The figure shows three views and two pictorial views of one solid part (mm, origin at its lowest corner). Answer the questions. A direction names the side the tool comes from. Round coordinates to 2 decimals unless told otherwise and drop trailing zeros. Write each loop counter-clockwise with the first axis right and the second up, starting at its lowest first coordinate (ties: lowest second). Pieces come first, ordered by that corner, then holes.
Item 1: A tool of negligible diameter and unlimited length cuts with its end or side. For the marked faces 1 and 2, from which of +Z, -Z, +X, -X, +Y, -Y can it reach the whole face along a straight path? Write none if from no direction.
Item 2: Find section C-C on y = 37. Give the vertices of the cut face in (x, z).
Item 3: Each of these flat-tipped pins is pushed along its axis until it touches: pin 1 (10 mm diameter, centred on x = 52, z = 21.5, fed in from +Y); pin 2 (1 mm diameter, centred on x = 49, y = 43, fed in from -Z). Where does it stop, or does it pass through?
Item 4: Find the intervals of material crossed by probe 1 along X at (y, z) = (80, 2.5); probe 2 along Z at (x, y) = (13, 125.5), in increasing order.
Item 5: Find section A-A on y = 101.5. Give the vertices of the cut face in (x, z), then the cut area to 4 significant figures.
Item 6: Find section D-D on x = 55.5. Give the vertices of the cut face in (y, z).
Item 7: For a pull along X with two mould halves and no side action, classify the marked faces 3, 4, 5 and 6 as +X half, -X half, draft (parallel to the pull), parting line (faces both ways), or undercut.
Item 8: Find section B-B on z = 31. Give the vertices of the cut face in (x, y).
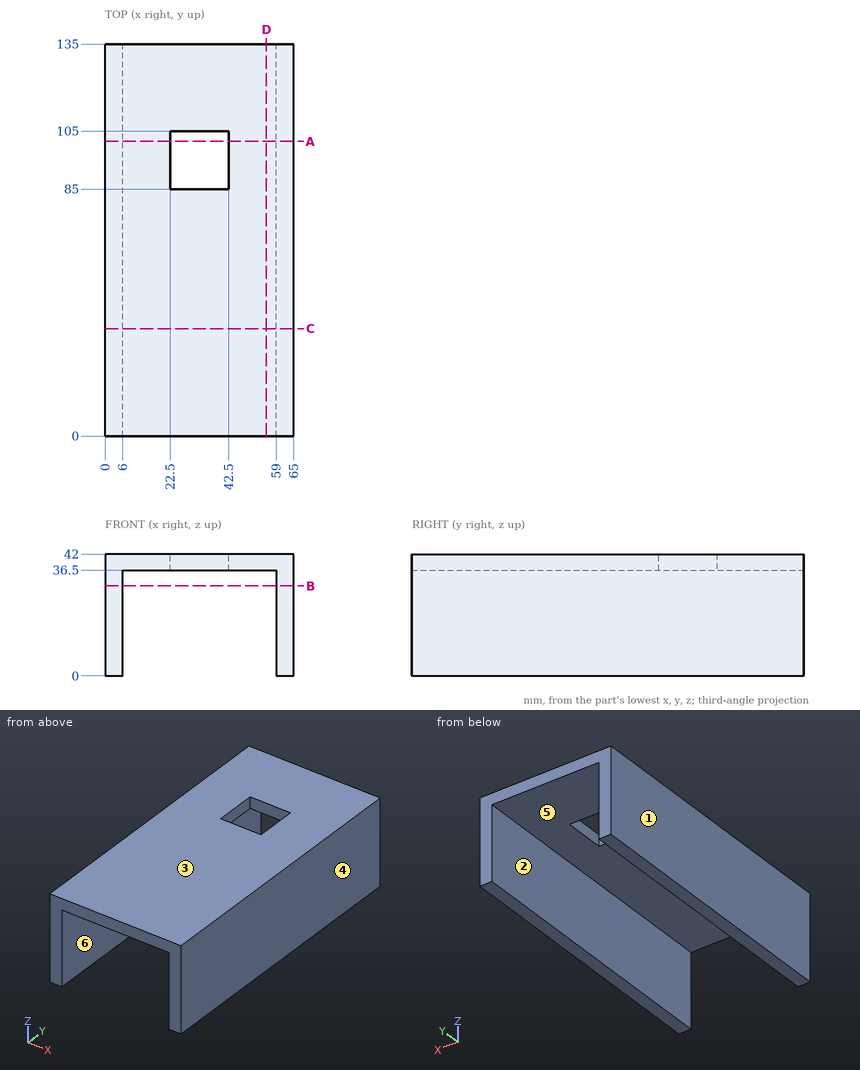
Check values:
1. face 1: +Z, -Z, -X, +Y, -Y
1. face 2: -Z, +Y, -Y
2. outline: (0, 0) - (6, 0) - (6, 36.5) - (59, 36.5) - (59, 0) - (65, 0) - (65, 42) - (0, 42) - close
3. pin 1: passes through
3. pin 2: stops at z = 36.5
4. probe 1: x = 0 to 6, 59 to 65
4. probe 2: z = 36.5 to 42
5. outline: (0, 0) - (6, 0) - (6, 36.5) - (22.5, 36.5) - (22.5, 42) - (0, 42) - close; (42.5, 36.5) - (59, 36.5) - (59, 0) - (65, 0) - (65, 42) - (42.5, 42) - close
5. area: 685.5 mm2
6. outline: (0, 36.5) - (135, 36.5) - (135, 42) - (0, 42) - close
7. face 3: draft
7. face 4: +X half
7. face 5: undercut
7. face 6: undercut
8. outline: (0, 0) - (6, 0) - (6, 135) - (0, 135) - close; (59, 0) - (65, 0) - (65, 135) - (59, 135) - close
